Source: three-view drawing plus pictorial views. Frame: mm from the lowest corner of the part. A direction names the side the tool comes from. Coordinates: 2 decimals unless noted, no trailing zeros. Loops run counter-clockwise (first coordinate to the right, second up) from the corner with the lowest first, then second, coordinate; pieces in that order, holes last. Notation, with made-up numbers: (-30.75, 70.5) - (4.25, 70.5) arc R11 cw to (4.25, 86.5) - close; hole circle Ø2 at (21, 2). An arc over 180 degrees is marked (long way). Return JSON: item names as keys, results as strings.
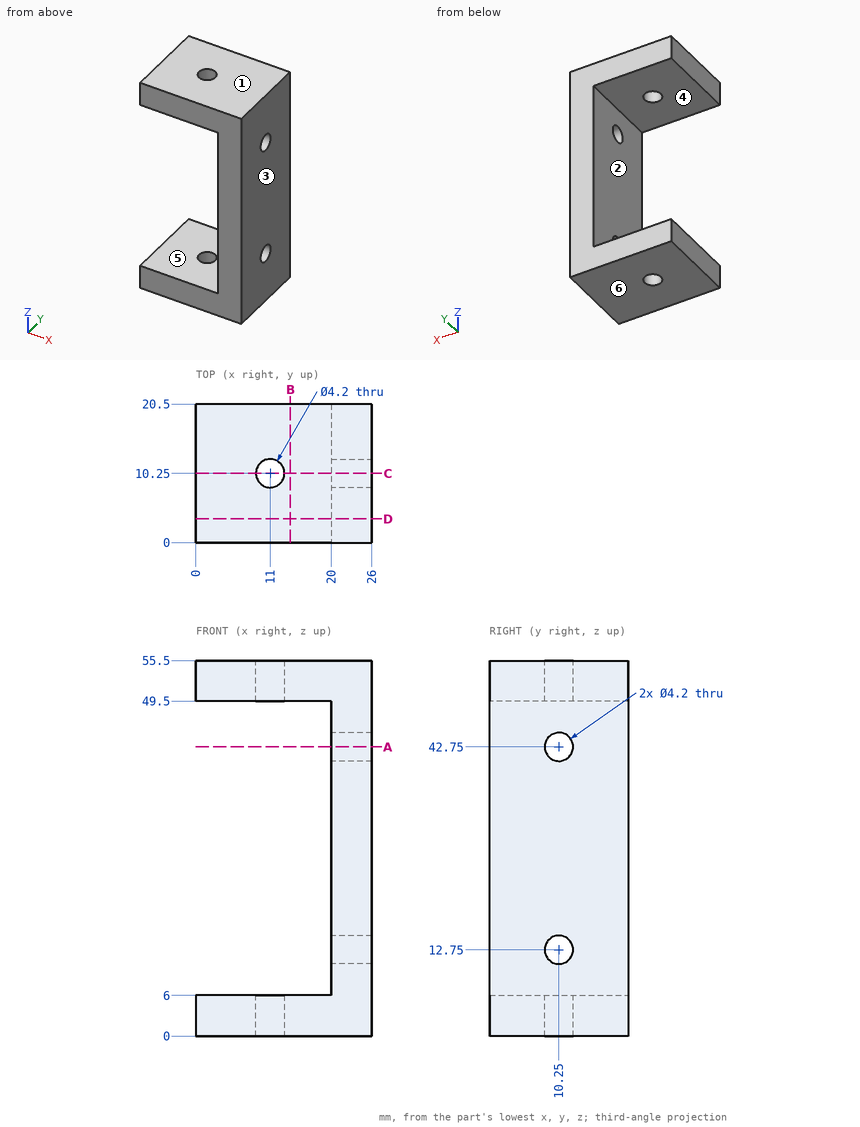
Item 1: Section query A-A, the plane z = 42.75. Return loops of the section in (x, y), and give its area (3 significant figures).
Worked out:
{"outline": "(20, 0) - (26, 0) - (26, 8.15) - (20, 8.15) - close; (20, 12.35) - (26, 12.35) - (26, 20.5) - (20, 20.5) - close", "area": "97.8 mm^2"}
Item 2: Section query B-B, the plane x = 14. Return loops of the section in (y, z), and give its area (3 significant figures).
Worked out:
{"outline": "(0, 0) - (20.5, 0) - (20.5, 6) - (0, 6) - close; (0, 49.5) - (20.5, 49.5) - (20.5, 55.5) - (0, 55.5) - close", "area": "246 mm^2"}
Item 3: Ray query, probe 1 along Z at (x, y) = (19.5, 4); probe 2 along Z at (x, y) = (23.75, 10.25); probe 3 along X at (y, z) = (16, 36). Return the intervals inside material, ascending. Write a range as from..to.
Worked out:
{"probe 1": "0..6, 49.5..55.5", "probe 2": "0..10.65, 14.85..40.65, 44.85..55.5", "probe 3": "20..26"}
Item 4: Section query C-C, the plane y = 10.25. Return loops of the section in (x, z), and give its area (3 significant figures).
Worked out:
{"outline": "(0, 0) - (8.9, 0) - (8.9, 6) - (0, 6) - close; (0, 49.5) - (8.9, 49.5) - (8.9, 55.5) - (0, 55.5) - close; (13.1, 0) - (26, 0) - (26, 10.65) - (20, 10.65) - (20, 6) - (13.1, 6) - close; (13.1, 49.5) - (20, 49.5) - (20, 44.85) - (26, 44.85) - (26, 55.5) - (13.1, 55.5) - close; (20, 14.85) - (26, 14.85) - (26, 40.65) - (20, 40.65) - close", "area": "472 mm^2"}
Item 5: Reachability of the marked faces 5 and 6 from +Z, -Z, +X, -X, +Y, -Y: full face, straight path, thin tool, end or side. Return the list, or none.
Worked out:
{"face 5": "-X, +Y, -Y", "face 6": "-Z, +X, -X, +Y, -Y"}
Item 6: First-contact query: pin 1 Ø1.5 at (y, z) = (14.5, 19) entering from -X. Flat tip, straight axial feed; report the tip coordinate or a pass-through.
Worked out:
{"pin 1": "x = 20"}
Item 7: Mould query, pull axis Z, two halves, no side actions, for the marked faces 1, 2, 3 and 4. Classes: +Z half, -Z half, draft (parallel to the pull), parting line (faces both ways), or undercut.
Worked out:
{"face 1": "+Z half", "face 2": "undercut", "face 3": "draft", "face 4": "undercut"}
Item 8: Section query D-D, the plane y = 3.5. Return loops of the section in (x, z).
Worked out:
{"outline": "(0, 0) - (26, 0) - (26, 55.5) - (0, 55.5) - (0, 49.5) - (20, 49.5) - (20, 6) - (0, 6) - close"}
